Autodesk Inventor part; units mm, degrees
ref_plane "YZ Plane" through (0, 0, 0) normal (1, 0, 0) x (0, 1, 0)
ref_plane "XZ Plane" through (0, 0, 0) normal (0, 1, 0) x (-1, 0, 0)
ref_plane "XY Plane" through (0, 0, 0) normal (0, 0, 1) x (1, 0, 0)
sketch "Sketch1" plane through (0, 0, 0) normal (0, 1, 0) x (-1, 0, 0)
  line L0 (0, 0) -> (50.8, 0)
  line L1 (50.8, 0) -> (50.8, -25.4)
  line L2 (50.8, -25.4) -> (0, -25.4)
  line L3 (0, -25.4) -> (0, 0)
  circle A0 centre (19.05, -12.7) radius 3.2639
  circle A1 centre (38.1, -12.7) radius 3.2639
  point P0 (0, -12.7)
  dimension "d0" = 50.8
  dimension "d1" = 25.4
  dimension "d2" = 6.5278
  dimension "d3" = 19.05
  dimension "d4" = 19.05
  dimension "d5" = 12.7
extrude "Extrusion1" add sketch "Sketch1" along normal blind 6.35
sketch "Sketch2" plane through (0, 6.35, 0) normal (0, 1, 0) x (1, 0, 0)
  line L0 (0, 25.4) -> (-50.8, 25.4)
  line L1 (0, 0) -> (-6.35, 0)
  line L2 (-6.35, 0) -> (-6.35, 25.4)
  line L3 (-6.35, 25.4) -> (0, 25.4)
  line L4 (0, 25.4) -> (0, 0)
  dimension "d8" = 6.35
extrude "Extrusion2" add sketch "Sketch2" along normal blind 63.5
sketch "Sketch3" plane through (-6.35, 6.35, -25.4) normal (-1, 0, 0) x (0, 0, 1)
  circle A0 centre (12.7, 12.7) radius 2.4892
  circle A1 centre (12.7, 38.1) radius 2.4892
  line L0 (0, 0) -> (25.4, 0)
  line L1 (25.4, 0) -> (25.4, 63.5)
  circle A2 centre (12.7, 50.8) radius 2.4892
  circle A3 centre (12.7, 25.4) radius 2.4892
  point P0 (25.4, -6.35)
  dimension "d11" = 4.9784
  dimension "d12" = 4.9784
  dimension "d13" = 25.4
  dimension "d14" = 12.7
  dimension "d15" = 12.7
  dimension "d23" = 12.7
  dimension "d24" = 12.7
extrude "Extrusion3" cut sketch "Sketch3" against normal through all
sketch "Sketch4" plane through (-50.8, 0, 0) normal (0, 0, 1) x (1, 0, 0)
  line L0 (0, 6.35) -> (44.45, 6.35)
  line L1 (0, 0) -> (50.8, 0)
  line L2 (50.8, 0) -> (50.8, 69.85)
  line L3 (44.45, 69.85) -> (50.8, 69.85)
  line L4 (44.45, 6.35) -> (44.45, 69.85)
  line L5 (0, 6.35) -> (44.45, 6.35)
  line L6 (0, 0) -> (0, 6.35)
  line L7 (0, 6.35) -> (44.45, 69.85)
  line L8 (50.8, 69.85) -> (50.8, 0)
  line L9 (0, 0) -> (0, 6.35)
  line L10 (50.8, 0) -> (0, 0)
  line L11 (44.45, 69.85) -> (50.8, 69.85)
extrude "Extrusion4" add sketch "Sketch4" against normal blind 3.175 contours L7 L4 L0
sketch "Sketch5" plane through (0, 0, -25.4) normal (0, 0, -1) x (-1, 0, 0)
  line L0 (0, 0) -> (50.8, 0)
  line L1 (50.8, 0) -> (50.8, 6.35)
  line L2 (6.35, 6.35) -> (50.8, 6.35)
  line L3 (6.35, 6.35) -> (6.35, 69.85)
  line L4 (0, 69.85) -> (6.35, 69.85)
  line L5 (0, 0) -> (0, 69.85)
  line L6 (50.8, 6.35) -> (50.8, 0)
  line L7 (0, 0) -> (50.8, 0)
  line L8 (50.8, 6.35) -> (6.35, 69.85)
  line L9 (0, 0) -> (0, 69.85)
  line L10 (6.35, 69.85) -> (0, 69.85)
  line L11 (0, 69.85) -> (0, 0)
extrude "Extrusion5" add sketch "Sketch5" against normal blind 3.175
fillet "Fillet1" radius 6.35 2 edges at (-50.8, 3.175, -25.4) (-50.8, 3.175, 0)
properties part number "INDX_005_Cornerbracket" material "ABS Plastic"
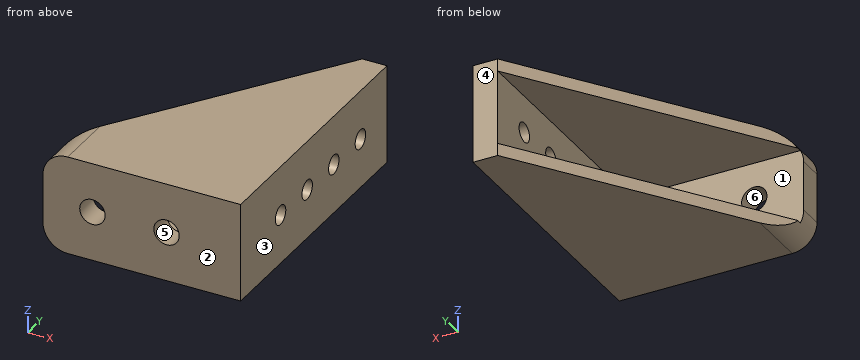
Geometry check sheet. Reference: the model listing, model coordinates, mm. Face numbers are marked on the shaded views. A direction names the side the tool comes from. Coordinates: 2 decimals unless noted, no trailing zeros. Order: outer loops, then holes, each group sorted by start corner. A loop starts at its lowest first (then second) coordinate and runs counter-clockwise, first axis right, second up. Notation, with made-up numbers: (23.25, 45) - (28.25, 45) arc R10 cw to (28.25, 53) - close; hole circle Ø3 at (19.25, -16.75). An arc over 180 degrees is marked (long way). One line per item, written item: value.
(1) Thickness scan on probe 1 along Y at (x, z) = (-3.75, -12.7); probe 2 along Z at (x, y) = (-19.05, 5); probe 3 along Z at (x, y) = (-17.5, 18) (3 decimals). Record the ranges inside material, lowest first. Write a range as from..to.
Data:
probe 1: y = 0..16.56, 21.54..29.26, 34.24..41.96, 46.94..54.66, 59.64..69.85
probe 2: z = -25.4..-15.96, -9.44..0
probe 3: z = -25.4..-22.225, -3.175..0
(2) Sectioned sample at C-C (x = -19.05). Enter the section's corners in (y, z) (3 decimals), and give its area (3 significant figures).
Data:
outline: (0, -25.4) - (51.707, -25.4) - (51.707, -22.225) - (6.35, -22.225) - (6.35, -15.964) - (0, -15.964) - close; (0, -9.436) - (6.35, -9.436) - (6.35, -3.175) - (51.707, -3.175) - (51.707, 0) - (0, 0) - close
area: 408 mm^2
(3) Sectioned sample at A-A (y = 44.45). Enter the section's corners in (x, z) (3 decimals).
Data:
outline: (-24.13, -25.4) - (0, -25.4) - (0, -15.189) - (-6.35, -15.189) - (-6.35, -22.225) - (-24.13, -22.225) - close; (-24.13, -3.175) - (-6.35, -3.175) - (-6.35, -10.211) - (0, -10.211) - (0, 0) - (-24.13, 0) - close
(4) Access from +Z, -Z, +X, -X, +Y, -Y to the whole of each face (thin tool, end or side, straight path). Record for the marked faces 1 and 2.
Data:
face 1: -X, +Y
face 2: +Z, -Z, +X, -X, -Y
(5) Release check for a two-part mould opening along X. For the marked faces 3, 4, 5 and 6 record: +X half, -X half, draft (parallel to the pull), parting line (faces both ways), or undercut.
Data:
face 3: +X half
face 4: draft
face 5: undercut
face 6: undercut
(6) Sectioned sample at D-D (z = -13.5). Count the separate pieces of the cut face and the enclosed holes in it, and give its area (3 significant figures).
Data:
separate pieces: 7
enclosed holes: 0
area: 526 mm^2
(7) Depth check by flat-ended pin: pin 1 Ø5.5 at (y, z) = (31.5, -8) entering from -X; pin 2 Ø10 at (x, z) = (-28, -14) entering from +Y. Enter the tip coordinate at first touch or a pass-through.
Data:
pin 1: stops at x = -6.35
pin 2: stops at y = 6.35
(8) Sectioned sample at B-B (x = -3.5). Enter the section's corners in (y, z), and give its area (3 significant figures).
Data:
outline: (0, -25.4) - (69.85, -25.4) - (69.85, 0) - (0, 0) - close; hole circle Ø4.98 at (19.05, -12.7); hole circle Ø4.98 at (31.75, -12.7); hole circle Ø4.98 at (44.45, -12.7); hole circle Ø4.98 at (57.15, -12.7)
area: 1,700 mm^2
